Here's how the part is built. I have some questions about the finished solid (model axes, mm). A direction names the side the tool comes from. Round coordinates to 2 decimals unless told otherwise and drop trailing zeros. Order: outer loops, then holes, each group sorted by start corner. A loop starts at its lowest first (then second) coordinate and runs counter-clockwise, first axis right, second up. Notation, with made-up numbers: (36.5, 57) -> (42.5, 57) arc R26 ccw to (42.5, 82) -> close; hole circle Ø4 at (17.25, 41). An arc over 180 degrees is marked (long way). Answer in a Markdown table with one row per item.
```python
from build123d import *

# Parameters (mm, degrees)
SKETCH1_R           = 2.159
SKETCH1_R_2         = 1.7272
SKETCH1_R_3         = 3.429
SKETCH1_W           = 40.894
SKETCH1_H           = 20.32
BOSS_EXTRUDE1_DEPTH = 3.2004
CUT_EXTRUDE1_DEPTH  = 3.2004
FILLET1_R           = 0.762


with BuildPart() as part:
    # Sketch1 → Boss-Extrude1 (new body)
    with BuildSketch(Plane.XY):
        Polygon((0, 0), (44.45, 0), (44.45, 25.4), (51.435, 25.4), (51.435, 53.464659022), (-6.985, 53.464659022), (-6.985, 25.4), (0, 25.4), align=None)
        with Locations((9.525, 12.7)):
            Circle(SKETCH1_R, mode=Mode.SUBTRACT)
        with Locations((34.925, 12.7)):
            Circle(SKETCH1_R, mode=Mode.SUBTRACT)
        with Locations((47.475, 34.131115311)):
            Circle(SKETCH1_R_2, mode=Mode.SUBTRACT)
        with Locations((-3.025, 44.131115311)):
            Circle(SKETCH1_R_2, mode=Mode.SUBTRACT)
        with Locations((-3.025, 34.131115311)):
            Circle(SKETCH1_R_2, mode=Mode.SUBTRACT)
        with Locations((47.475, 44.131115311)):
            Circle(SKETCH1_R_2, mode=Mode.SUBTRACT)
        with Locations((22.225, 17.4625)):
            Circle(SKETCH1_R_3, mode=Mode.SUBTRACT)
        with Locations((22.225, 7.9375)):
            Circle(SKETCH1_R, mode=Mode.SUBTRACT)
        with Locations((22.225, 39.131115311)):
            Rectangle(SKETCH1_W, SKETCH1_H, mode=Mode.SUBTRACT)
    extrude(amount=BOSS_EXTRUDE1_DEPTH)

    # Sketch2 → Cut-Extrude1 (cut)
    with BuildSketch(Plane.XY.offset(3.2004)):
        with BuildLine():
            Line((-2.286, 40.147115311), (1.778, 40.147115311))
            Line((1.778, 40.147115311), (1.778, 38.115115311))
            Line((1.778, 38.115115311), (-2.286, 38.115115311))
            ThreePointArc((-2.286, 38.115115311), (-3.302, 39.131115311), (-2.286, 40.147115311))
        make_face()
        with BuildLine():
            Line((42.672, 40.147115311), (46.736, 40.147115311))
            ThreePointArc((46.736, 40.147115311), (47.752, 39.131115311), (46.736, 38.115115311))
            Line((46.736, 38.115115311), (42.672, 38.115115311))
            Line((42.672, 38.115115311), (42.672, 40.147115311))
        make_face()
    extrude(amount=-CUT_EXTRUDE1_DEPTH, mode=Mode.SUBTRACT)

    # Fillet1
    fillet1_edges = [part.edges().sort_by_distance(p)[0] for p in [
        (51.435, 53.464659022, 1.6002),
        (51.435, 25.4, 1.6002),
        (44.45, 0, 1.6002),
        (0, 0, 1.6002),
        (-6.985, 25.4, 1.6002),
        (-6.985, 53.464659022, 1.6002),
    ]]
    fillet(fillet1_edges, radius=FILLET1_R)


solid = part.part
```
1. For faces 5 (the face through (-6.985, 40, 2)), 6 (the face through (48, 25.4, 2)), 7 (the face through (-3.3, 39.1, 1.6)), which set-ups out of +Z, -Z, +X, -X, +Y, -Y let a thin tool reach every point of the face, with its end or its side?
Numbers:
| item | result |
|---|---|
| face 5 | +Z, -Z, -X, +Y, -Y |
| face 6 | +Z, -Z, +X, -Y |
| face 7 | +Z, -Z |
2. Suppose I cut it at D-D on y = 45. Write out the boundary of the cut face in (x, z) (3 decimals), then the cut area to 3 significant figures.
Numbers:
| item | result |
|---|---|
| outline | (-6.985, 0) -> (-4.518, 0) -> (-4.518, 3.2) -> (-6.985, 3.2) -> close; (-1.532, 0) -> (1.778, 0) -> (1.778, 3.2) -> (-1.532, 3.2) -> close; (42.672, 0) -> (45.982, 0) -> (45.982, 3.2) -> (42.672, 3.2) -> close; (48.968, 0) -> (51.435, 0) -> (51.435, 3.2) -> (48.968, 3.2) -> close |
| area | 37.0 mm2 |
3. We'd pull the mould along X, two halves only. Please class faces 1 (the face through (47.75, 39.15, 1.62)), 2 (the face through (36.92, 11.87, 1.58)), 3 (the face through (51.435, 39, 2)), 4 (the face through (-3, 25.4, 2)): released by +X, released by -X, zero draft, split by the parting line, or undercut.
Numbers:
| item | result |
|---|---|
| face 1 | undercut |
| face 2 | undercut |
| face 3 | released by +X |
| face 4 | zero draft |
4. For pin 1 Ø1 at (x, z) = (-4, 2) entering from -Y, with a flat end and sliding along its axis, tell me the tip position at first contact or that it passes through.
Numbers:
| item | result |
|---|---|
| pin 1 | stops at y = 25.4 |
5. Suppose I cut it at B-B on x = 6. Write out the boundary of the cut face in (y, z), then the cut area to 3 significant figures.
Numbers:
| item | result |
|---|---|
| outline | (0, 0) -> (28.97, 0) -> (28.97, 3.2) -> (0, 3.2) -> close; (49.29, 0) -> (53.46, 0) -> (53.46, 3.2) -> (49.29, 3.2) -> close |
| area | 106 mm2 |
6. Suppose I cut it at A-A on y = 12.7. Write out the boundary of the cut face in (x, z), then the cut area to 3 significant figures.
Numbers:
| item | result |
|---|---|
| outline | (0, 0) -> (7.37, 0) -> (7.37, 3.2) -> (0, 3.2) -> close; (11.68, 0) -> (32.77, 0) -> (32.77, 3.2) -> (11.68, 3.2) -> close; (37.08, 0) -> (44.45, 0) -> (44.45, 3.2) -> (37.08, 3.2) -> close |
| area | 115 mm2 |
7. Suppose I cut it at C-C on z = 1.85. State how many separate pieces and enclosed holes the cut face has, then the cut area to 3 significant figures.
Numbers:
| item | result |
|---|---|
| separate pieces | 1 |
| enclosed holes | 9 |
| area | 1,800 mm2 |
8. Please list where these lines run through material, in increasing order: line 1 along X through (y, z) = (12.5, 3.05); line 2 along Y through (x, z) = (43.5, 2.8); line 3 along Y through (x, z) = (29.5, 1.9).
Numbers:
| item | result |
|---|---|
| line 1 | x = 0 to 7.38, 11.67 to 32.78, 37.07 to 44.45 |
| line 2 | y = 0 to 38.12, 40.15 to 53.46 |
| line 3 | y = 0 to 28.97, 49.29 to 53.46 |
